Autodesk Inventor part; units mm, degrees
ref_plane "YZ Plane" through (0, 0, 0) normal (1, 0, 0) x (0, 1, 0)
ref_plane "XZ Plane" through (0, 0, 0) normal (0, 1, 0) x (-1, 0, 0)
ref_plane "XY Plane" through (0, 0, 0) normal (0, 0, 1) x (1, 0, 0)
sketch "Sketch2" plane through (0, 0, 0) normal (1, 0, 0) x (0, 1, 0)
  line L0 (0, 0) -> (70, 0)
  line L1 (0, 0) -> (0, -305)
  line L2 (0, -305) -> (20, -305)
  line L3 (20, -305) -> (70, 0)
  dimension "d2" = 70
  dimension "d3" = 305
  dimension "d4" = 20
extrude "Extrusion1" add sketch "Sketch2" along normal blind 40
sketch "Sketch3" plane through (0, 0, 0) normal (0, 0, 1) x (1, 0, 0)
  line L0 (0, 35) -> (40, 35)
  line L1 (0, 0) -> (40, 0)
  line L2 (20, 0) -> (20, 70)
  line L3 (0, 70) -> (40, 70)
  circle A0 centre (20, 35) radius 10
  dimension "d7" = 35
  dimension "d8" = 20
extrude "Extrusion2" cut sketch "Sketch3" against normal blind 52
properties part number "Car Base" material "Wood (Maple)"
Read the model definition and answer for the solid it produces. Units are mm, in the model's axes. A direction names the side the tool comes from. Give positions to 0.01 mm unless a question says otherwise; leave off trailing zeros. Write each loop counter-clockwise with the first axis right and the second up, starting at its lowest first coordinate (ties: lowest second). Pieces come first, ordered by that corner, then holes. Notation, with made-up numbers: M 29.5,-19 L 43.5,-19 A22 cw 43.5,5 Z; hole C 77.25,1.25 d6. An arc over 180 degrees is marked long. Put each result on its own line as item: value. Start each with the question number.
1. For a pull along X with two mould halves and no side action, classify faces 3 (the flat face through (0, 27, -116)), 4 (the flat face through (20, 10, -305)), 5 (the flat face through (20, 35, -52)) as released by +X, released by -X, zero draft, split by the parting line, or undercut.
2. The part is cut by section A-A, the plane x = 20. Give the vertices of the cut face in (y, z).
3. Each of these flat-tipped pins is pushed along its axis until it touches: pin 1 Ø1.5 at (y, z) = (34.5, -228) entering from -X; pin 2 Ø2 at (x, z) = (10, -74.5) entering from +Y. Where does it stop, or does it pass through?
4. Which of the six approach directions +Z, -Z, +X, -X, +Y, -Y give full straight-line access (tool end or side, diameter ignored) to faces 1 (the flat face through (19.72, 44.65, -154.63)), 2 (the cylindrical face through (24.614, 26.128, -25.636))?
5. The part is cut by section C-C, the plane z = -22. Give the vertices of the cut face in (x, y), and give its area (3 significant figures).
6. The part is cut by section B-B, the plane y = 35. Give the vertices of the cut face in (x, z), and give its area (3 significant figures).
7. The part is cut by section D-D, the plane z = -244. Give the vertices of the cut face in (x, y).
8. Consider line 1 along X through (y, z) = (35, -38.5); line 2 along Y through (x, z) = (20, -11.5); line 3 along Y through (x, z) = (20, -19). Determine where each line is inside the solid, lowest interval first.
Final values:
1. face 3: released by -X
1. face 4: zero draft
1. face 5: undercut
2. outline: M 0,-305 L 20,-305 L 70,0 L 45,0 L 45,-52 L 25,-52 L 25,0 L 0,0 Z
3. pin 1: passes through
3. pin 2: stops at y = 57.95
4. face 1: -Z, +X, -X, +Y
4. face 2: +Z
5. outline: M 0,0 L 40,0 L 40,66.39 L 0,66.39 Z; hole C 20,35 d20
5. area: 2,340 mm²
6. outline: M 0,-213.5 L 40,-213.5 L 40,0 L 30,0 L 30,-52 L 10,-52 L 10,0 L 0,0 Z
6. area: 7,500 mm²
7. outline: M 0,0 L 40,0 L 40,30 L 0,30 Z
8. line 1: x = 0 to 10, 30 to 40
8. line 2: y = 0 to 25, 45 to 68.11
8. line 3: y = 0 to 25, 45 to 66.89
